Read the model definition and answer for the solid it produces. Units are mm, in the model's axes. Face numbers are marked on the shaded views. Coordinates: 2 decimals unless noted, no trailing zeros. Write each loop counter-clockwise with the first axis right and the second up, starting at its lowest first coordinate (ties: lowest second). Pieces come first, ordered by that corner, then holes.
1) The part is cut by section B-B (y = 0). Determine the outline of the cut face in (x, z), then the cut area to 3 significant figures.
2) The part is cut by section D-D (x = 0). Determine the outline of the cut face in (y, z).
3) The part is cut by section C-C (z = -0.5). Give the number of separate pieces and of enclosed holes in the cut face, then the cut area to 3 significant figures.
4) Find the intervals of material crossed by line 1 (X direction, y = 1.7, z = 0); line 2 (Z direction, x = -1.5, y = -1.35); line 3 (Y direction, x = 9.5, z = 0), in increasing order.
5) The part is cut by section A-A (x = -7.5). Determine the outline of the cut face in (y, z), then the cut area to 3 significant figures.
6) Determine the mould class of the marked faces 1, 2, 3 and 4 for opening direction Y: +Y half, -Y half, draft (parallel to the pull), parting line (faces both ways), or undercut.
from build123d import *

# Parameters (mm, degrees)
SKETCH_1_W          = 24
SKETCH_1_H          = 5
EXTRUDE_1_DEPTH     = 3
SKETCH_2_R          = 1.5
CUT_EXTRUDE_1_DEPTH = 25.315632832
SKETCH_3_R          = 1.75
CUT_EXTRUDE_2_DEPTH = 14.341664064
SKETCH_4_R          = 1
CUT_EXTRUDE_3_DEPTH = 14.341664192
SKETCH_5_R          = 1
EXTRUDE_3_DEPTH     = 2
SKETCH_6_W          = 2
SKETCH_6_H          = 0.5
CUT_EXTRUDE_7_DEPTH = 3
CUT_EXTRUDE_START   = -10
SKETCH_8_R          = 1
CUT_EXTRUDE_9_DEPTH = 10
FILLET_2_R          = 2


with BuildPart() as part:
    # 草图1 → 凸台-拉伸1 (new, symmetric)
    with BuildSketch(Plane.XY):
        Rectangle(SKETCH_1_W, SKETCH_1_H)
    extrude(amount=EXTRUDE_1_DEPTH, both=True)

    # 草图2 → 切除-拉伸1 (cut, through all)
    with BuildSketch(Plane(origin=(12, 0, 0), x_dir=(0, 0, -1), z_dir=(1, 0, 0))):
        Circle(SKETCH_2_R)
    extrude(amount=-CUT_EXTRUDE_1_DEPTH, mode=Mode.SUBTRACT)

    # 草图3 → 切除-拉伸2 (cut, through all)
    with BuildSketch(Plane(origin=(0, 2.5, 0), x_dir=(1, 0, 0), z_dir=(0, 1, 0))):
        with Locations(Location((0, 0, 0), (0, 0, 270))):
            Circle(SKETCH_3_R)
    extrude(amount=-CUT_EXTRUDE_2_DEPTH, mode=Mode.SUBTRACT)

    # 草图4 → 切除-拉伸3 (cut, through all)
    with BuildSketch(Plane(origin=(0, 2.5, 0), x_dir=(1, 0, 0), z_dir=(0, 1, 0))):
        with Locations(Location((-7, 0, 0), (0, 0, 270))):
            Circle(SKETCH_4_R)
    extrude(amount=-CUT_EXTRUDE_3_DEPTH, mode=Mode.SUBTRACT)

    # 草图5 → 凸台-拉伸3 (add)
    with BuildSketch(Plane(origin=(0, 2.5, 0), x_dir=(1, 0, 0), z_dir=(0, 1, 0))):
        with Locations(Location((7, 0, 0), (0, 0, 270))):
            Circle(SKETCH_5_R)
    extrude(amount=EXTRUDE_3_DEPTH)

    # 草图6 → 切除-拉伸7 (cut)
    with BuildSketch(Plane(origin=(0, 0, -3), x_dir=(-1, 0, 0), z_dir=(0, 0, -1))):
        with Locations((-7, 3.25)):
            Rectangle(SKETCH_6_W, SKETCH_6_H)
    extrude(amount=-CUT_EXTRUDE_7_DEPTH, mode=Mode.SUBTRACT)

    # 草图8 → 切除-拉伸9 (cut)
    with BuildSketch(Plane(origin=(0, 4.5, 0), x_dir=(1, 0, 0), z_dir=(0, 1, 0)).offset(CUT_EXTRUDE_START)):
        with Locations(Location((7, 0, 0), (0, 0, 270))):
            Circle(SKETCH_8_R)
    extrude(amount=CUT_EXTRUDE_9_DEPTH, mode=Mode.SUBTRACT)

    # 圆角2
    # the kernel refuses this fillet: 2 mm, written as the material it takes off along each edge
    with BuildSketch(Plane(origin=(17, 2.5, -3), x_dir=(0, -1, 0), z_dir=(-1, 0, 0))) as fillet_2_piece_1:
        with BuildLine():
            CenterArc((FILLET_2_R, FILLET_2_R), FILLET_2_R, 180, 90)
            Line((0, FILLET_2_R), (0, 0))
            Line((0, 0), (FILLET_2_R, 0))
        make_face()
    extrude(amount=34, mode=Mode.SUBTRACT)
    with BuildSketch(Plane(origin=(17, 2.5, 3), x_dir=(0, -1, 0), z_dir=(-1, 0, 0))) as fillet_2_piece_2:
        with BuildLine():
            CenterArc((FILLET_2_R, -FILLET_2_R), FILLET_2_R, 90, 90)
            Line((0, -FILLET_2_R), (0, 0))
            Line((0, 0), (FILLET_2_R, 0))
        make_face()
    extrude(amount=34, mode=Mode.SUBTRACT)


solid = part.part
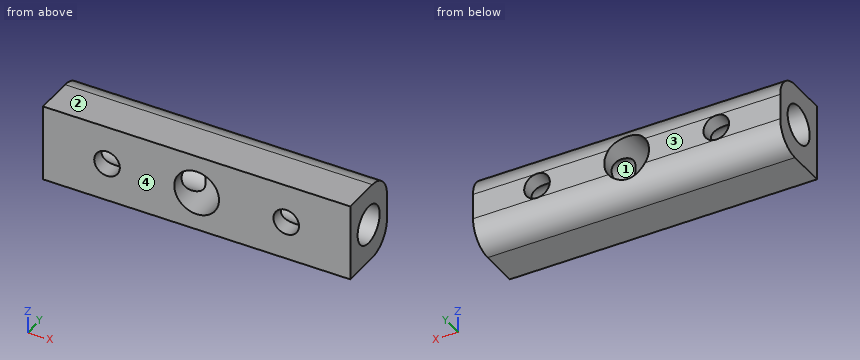
Reported:
1. outline: (-12, -3) - (12, -3) - (12, -1.5) - (0.9, -1.5) arc R1.75 cw to (-0.9, -1.5) - (-12, -1.5) - close; (-12, 1.5) - (-0.9, 1.5) arc R1.75 cw to (0.9, 1.5) - (12, 1.5) - (12, 3) - (-12, 3) - close
1. area: 71.4 mm2
2. outline: (-2.5, -3) - (0.5, -3) arc R2 ccw to (2.35, -1.75) - (-2.5, -1.75) - close; (-2.5, 1.75) - (2.35, 1.75) arc R2 ccw to (0.5, 3) - (-2.5, 3) - close
3. separate pieces: 8
3. enclosed holes: 0
3. area: 37.3 mm2
4. line 1: x = -12 to -8, -6 to -1.75, 1.75 to 6, 8 to 12
4. line 2: z = -3 to -0.9, 0.9 to 3
4. line 3: y = -2.5 to -1.5, 1.5 to 2.5
5. outline: (-2.5, -3) - (0.5, -3) arc R2 ccw to (2.5, -1) - (2.5, -0.87) - (1.22, -0.87) arc R1.5 cw to (-1.22, -0.87) - (-2.5, -0.87) - close; (-2.5, 0.87) - (-1.22, 0.87) arc R1.5 cw to (1.22, 0.87) - (2.5, 0.87) - (2.5, 1) arc R2 ccw to (0.5, 3) - (-2.5, 3) - close
5. area: 17.4 mm2
6. face 1: undercut
6. face 2: draft
6. face 3: +Y half
6. face 4: -Y half
